Here's how the part is built. I have some questions about the finished solid (model axes, mm). A direction names the side the tool comes from. Round coordinates to 2 decimals unless told otherwise and drop trailing zeros. Loops run counter-clockwise (first coordinate to the right, second up) from the corner with the lowest first, then second, coordinate; pieces in that order, holes last. Notation, with made-up numbers: M -40,12 L 3,12 A19 cw 3,35 Z; hole C 6.25,-17.5 d11. An arc over 180 degrees is marked long. Use a Markdown table: item, result.
```python
from build123d import *

# Parameters (mm, degrees)
F0_R     = 2.35
F1_DEPTH = 70


with BuildPart() as f1:
    # F0 (on Front) → F1 (new body)
    with BuildSketch(Plane.XZ):
        with BuildLine():
            ThreePointArc((0.5, -3.312476), (0, -3.35), (-0.5, -3.312476))
            Line((-0.5, -3.312476), (-0.5, -6.312476))
            Line((-0.5, -6.312476), (0.5, -6.312476))
            Line((0.5, -6.312476), (0.5, -3.312476))
        make_face()
        with BuildLine():
            Line((0.5, -3.312476), (-0.5, -3.312476))
            ThreePointArc((-0.5, -3.312476), (0, -3.35), (0.5, -3.312476))
        make_face()
        with BuildLine():
            ThreePointArc((0.5, -3.312476), (2.539439, -2.184891), (3.35, 0))
            ThreePointArc((3.35, 0), (-2.184891, 2.539439), (-0.5, -3.312476))
            Line((-0.5, -3.312476), (0.5, -3.312476))
        make_face()
        Circle(F0_R, mode=Mode.SUBTRACT)
        Polygon((0.5, -6.312476), (-0.5, -6.312476), (-1.705153, -6.910453), (1.628228, -6.910453), align=None)
    extrude(amount=F1_DEPTH)


solid = f1.part
```
Q1. Imagine slicing it at A-A, the plane z = -1.75. Please give me the cut outline in (x, y).
Return value:
| item | result |
|---|---|
| outline | M -2.86,-70 L -1.57,-70 L -1.57,0 L -2.86,0 Z; M 1.57,-70 L 2.86,-70 L 2.86,0 L 1.57,0 Z |
Q2. Will these pins go through, and if not, where does the flat tip stop? P1, Ø2.5, axis at y = -18.5, z = -5, coming from the -X side; P2, Ø3.5, axis at y = -25.5, z = -4, coming from the +X side.
Return value:
| item | result |
|---|---|
| P1 | stops at x = -0.5 |
| P2 | stops at x = 2.48 |
Q3. For faces 4 (the flat face through (1.072, -34.51, -6.616)), 5 (the flat face through (-1.094, -34.51, -6.607)), 6 (the flat face through (0, -35, -6.91)), which set-ups out of +Z, -Z, +X, -X, +Y, -Y let a thin tool reach every point of the face, with its end or its side?
Return value:
| item | result |
|---|---|
| face 4 | +X, +Y, -Y |
| face 5 | -X, +Y, -Y |
| face 6 | -Z, +X, -X, +Y, -Y |
Q4. I need wall thicknesses on line 1 (Z direction, x = 0, y = -55.5); line 2 (Z direction, x = 1, y = -14); line 3 (X direction, y = -54.5, z = -0.25). Which ranges of each line are inside material? Lowest first, please. Write a range as from..to.
Return value:
| item | result |
|---|---|
| line 1 | z = -6.91..-2.35, 2.35..3.35 |
| line 2 | z = -6.91..-6.58, -3.2..-2.13, 2.13..3.2 |
| line 3 | x = -3.34..-2.34, 2.34..3.34 |
Q5. We'd pull the mould along X, two halves only. Please class faces 1 (the cylindrical face through (-0.509, -34.51, -2.294)), 2 (the flat face through (0, 0, -3)), 3 (the flat face through (0.5, -35, -5)): pulls with the +X half, pulls with the -X half, needs draft (parallel to the pull), parting line crosses it, or undercut.
Return value:
| item | result |
|---|---|
| face 1 | undercut |
| face 2 | needs draft |
| face 3 | pulls with the +X half |
Q6. Imagine slicing it at B-B, the plane y = -59. Please give me the cut outline in (x, z), then the cut area to 3 significant figures.
Return value:
| item | result |
|---|---|
| outline | M -1.71,-6.91 L 1.63,-6.91 L 0.5,-6.31 L 0.5,-3.31 A3.35 ccw long -0.5,-3.31 L -0.5,-6.31 Z; hole C 0,0 d4.7 |
| area | 22.2 mm^2 |
